from build123d import *

# Parameters (mm, degrees)
BOSS_EXTRUDE1_DEPTH = 133.35
SKETCH3_OUTSIDE_W   = 35.09
SKETCH3_OUTSIDE_H   = 36.072
SKETCH3_OUTSIDE_R   = 3.048
CUT_EXTRUDE1_DEPTH  = 57.15
SKETCH4_OUTSIDE_W   = 35.09
SKETCH4_OUTSIDE_H   = 36.072
SKETCH4_OUTSIDE_R   = 3.048
CUT_EXTRUDE2_DEPTH  = 15.875
SKETCH5_OUTSIDE_W   = 35.09
SKETCH5_OUTSIDE_H   = 36.072
SKETCH5_OUTSIDE_R   = 2.667
CUT_EXTRUDE3_DEPTH  = 1.6002


with BuildPart() as part:
    # Sketch2 → Boss-Extrude1 (new body)
    with BuildSketch(Plane.XY):
        Polygon((0, 3.666174209), (-3.175, 1.833087105), (-3.175, -1.833087105), (0, -3.666174209), (3.175, -1.833087105), (3.175, 1.833087105), align=None)
    extrude(amount=BOSS_EXTRUDE1_DEPTH)

    # Sketch3 outside → Cut-Extrude1 (cut)
    with BuildSketch(Plane.XY.offset(133.35)):
        Rectangle(SKETCH3_OUTSIDE_W, SKETCH3_OUTSIDE_H)
        Circle(SKETCH3_OUTSIDE_R, mode=Mode.SUBTRACT)
    extrude(amount=-CUT_EXTRUDE1_DEPTH, mode=Mode.SUBTRACT)

    # Sketch4 outside → Cut-Extrude2 (cut)
    with BuildSketch(Plane(origin=(0, 0, 0), x_dir=(-1, 0, 0), z_dir=(0, 0, -1))):
        Rectangle(SKETCH4_OUTSIDE_W, SKETCH4_OUTSIDE_H)
        Circle(SKETCH4_OUTSIDE_R, mode=Mode.SUBTRACT)
    extrude(amount=-CUT_EXTRUDE2_DEPTH, mode=Mode.SUBTRACT)

    # Sketch5 outside → Cut-Extrude3 (cut)
    with BuildSketch(Plane.XY.offset(131.064)):
        Rectangle(SKETCH5_OUTSIDE_W, SKETCH5_OUTSIDE_H)
        Circle(SKETCH5_OUTSIDE_R, mode=Mode.SUBTRACT)
    extrude(amount=-CUT_EXTRUDE3_DEPTH, mode=Mode.SUBTRACT)


solid = part.part
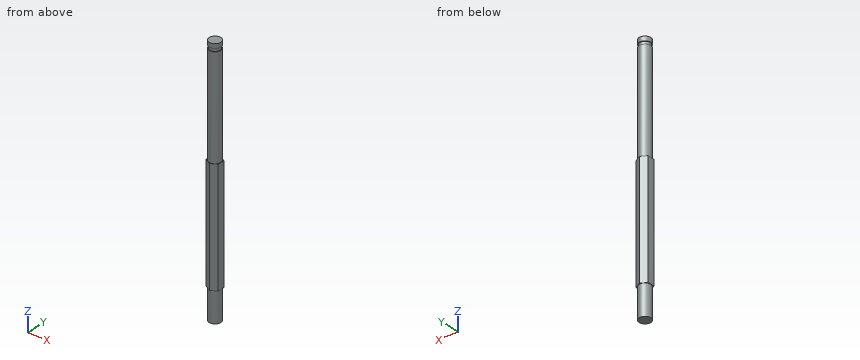
Part model, mm, in its own coordinate system. Give positions to 0.01 mm unless a question says otherwise; leave off trailing zeros. Write each loop counter-clockwise with the first axis right and the second up, starting at its lowest first coordinate (ties: lowest second). Pieces come first, ordered by that corner, then holes.
1) Pin check, flat tips, straight feed: pin 1 (1.5 mm diameter, centred on x = -0.5, z = 25.5, fed in from -Y); pin 2 (3 mm diameter, centred on x = 0.5, z = 82.5, fed in from -Y); pin 3 (1.5 mm diameter, centred on y = 0, z = 14.5, fed in from +X); pin 4 (3 mm diameter, centred on x = 1, y = 1, fed in from -Z). Stop position of each tip, or through.
Resolved:
pin 1: stops at y = -3.67
pin 2: stops at y = -3.05
pin 3: stops at x = 3.05
pin 4: stops at z = 0
2) Probe L1, parallel to Z at x = -2.25, y = 1.5; L2, parallel to Y at x = -1.5, z = 118; L3, parallel to Z at x = 2.75, y = -2 (3 decimals). List the from-to ranges inside material, lowest first.
Resolved:
L1: z = 0 to 129.46, 131.06 to 133.35
L2: y = -2.65 to 2.65
L3: z = 15.875 to 76.2
3) Cut at B-B on z = 110.5. Write the cut outline in (x, y), then the cut area to 3 significant figures.
Resolved:
outline: circle Ø6.1 at (0, 0)
area: 29.2 mm2
4) Cut at D-D on z = 71. Write the cut outline in (x, y) (3 decimals).
Resolved:
outline: (-3.175, -1.833) - (0, -3.666) - (3.175, -1.833) - (3.175, 1.833) - (0, 3.666) - (-3.175, 1.833) - close
5) Cut at A-A on y = 0. Write the cut outline in (x, z) (3 decimals).
Resolved:
outline: (-3.175, 15.875) - (-3.048, 15.875) - (-3.048, 0) - (3.048, 0) - (3.048, 15.875) - (3.175, 15.875) - (3.175, 76.2) - (3.048, 76.2) - (3.048, 129.464) - (2.667, 129.464) - (2.667, 131.064) - (3.048, 131.064) - (3.048, 133.35) - (-3.048, 133.35) - (-3.048, 131.064) - (-2.667, 131.064) - (-2.667, 129.464) - (-3.048, 129.464) - (-3.048, 76.2) - (-3.175, 76.2) - close
6) Cut at C-C on x = 1. Write the cut outline in (y, z) (3 decimals).
Resolved:
outline: (-3.089, 15.875) - (-2.879, 15.875) - (-2.879, 0) - (2.879, 0) - (2.879, 15.875) - (3.089, 15.875) - (3.089, 76.2) - (2.879, 76.2) - (2.879, 129.464) - (2.472, 129.464) - (2.472, 131.064) - (2.879, 131.064) - (2.879, 133.35) - (-2.879, 133.35) - (-2.879, 131.064) - (-2.472, 131.064) - (-2.472, 129.464) - (-2.879, 129.464) - (-2.879, 76.2) - (-3.089, 76.2) - close
